from build123d import *

# Parameters (mm, degrees)
SKETCH1_R           = 32.5
SKETCH1_R_2         = 29.5
BOSS_EXTRUDE1_DEPTH = 72
BOSS_EXTRUDE2_DEPTH = 72
CIRPATTERN1_COUNT   = 3
CIRPATTERN1_ANGLE   = 120
SKETCH7_R           = 12.5
BOSS_EXTRUDE5_DEPTH = 72
SKETCH9_R           = 9.9
CUT_EXTRUDE4_DEPTH  = 86.419552797


with BuildPart() as part:
    # Sketch1 → Boss-Extrude1 (new body)
    with BuildSketch(Plane.XY):
        Circle(SKETCH1_R)
        Circle(SKETCH1_R_2, mode=Mode.SUBTRACT)
    extrude(amount=BOSS_EXTRUDE1_DEPTH)

    # Sketch2 → Boss-Extrude2 (add, through all)
    with BuildSketch(Plane.XY):
        with BuildLine():
            Line((-29.461839725, -1.5), (29.461839725, -1.5))
            ThreePointArc((29.461839725, -1.5), (29.5, 0), (29.461839725, 1.5))
            Line((29.461839725, 1.5), (-29.461839725, 1.5))
            ThreePointArc((-29.461839725, 1.5), (-29.5, 0), (-29.461839725, -1.5))
        make_face()
    boss_extrude2 = extrude(amount=BOSS_EXTRUDE2_DEPTH)

    # CirPattern1: Boss-Extrude2 ×3 about axis
    cirpattern1_axis = Axis((0, 0, 0), (0, 0, 1))
    for i in range(1, CIRPATTERN1_COUNT):
        add(boss_extrude2.rotate(cirpattern1_axis, i * CIRPATTERN1_ANGLE / (CIRPATTERN1_COUNT - 1)))

    # Sketch7 → Boss-Extrude5 (add, through all)
    with BuildSketch(Plane.XY):
        Circle(SKETCH7_R)
    extrude(amount=BOSS_EXTRUDE5_DEPTH)

    # Sketch9 → Cut-Extrude4 (cut, through all)
    with BuildSketch(Plane.XY):
        Circle(SKETCH9_R)
    extrude(amount=CUT_EXTRUDE4_DEPTH, mode=Mode.SUBTRACT)


solid = part.part
Geometry: final body of the model. Coordinates: model frame, mm. Give positions to 0.01 mm unless a question says otherwise; leave off trailing zeros. Loops run counter-clockwise (first coordinate to the right, second up) from the corner with the lowest first, then second, coordinate; pieces in that order, holes last. Notation, with made-up numbers: (75.25, -27.5) -> (100.25, -27.5) arc R30 ccw to (100.25, 2.5) -> close; hole circle Ø11 at (84.25, 15.25). An arc over 180 degrees is marked (long way). Put each result on its own line as item: value.
1. Pin query (flat end, axial travel): P1, Ø4, axis at x = -21, z = 62.5, coming from the +Y side; P2, Ø1.5, axis at x = -20, z = 31.5, coming from the +Y side; P3, Ø12, axis at y = -15, z = 54.5, coming from the -X side. Return the tip coordinate at first contact, or that it passes through.
Taken from the geometry:
P1: stops at y = 26.37
P2: stops at y = 26.19
P3: stops at x = -31.23
2. Pull-direction query (X, two-part tool) for faces 1 (the flat face through (-11.827, 17.484, 35.496)), 2 (the flat face through (-10, -3, 0)), 3 (the cylindrical face through (31, 9.76, 35.5)); classes: released by +X, released by -X, zero draft, split by the parting line, or undercut.
Taken from the geometry:
face 1: undercut
face 2: zero draft
face 3: split by the parting line
3. Cut plane A-A (y = 15). Return the cut outline in (x, z).
Taken from the geometry:
outline: (-28.83, 0) -> (-25.4, 0) -> (-25.4, 72) -> (-28.83, 72) -> close; (-10.39, 0) -> (-6.93, 0) -> (-6.93, 72) -> (-10.39, 72) -> close; (6.93, 0) -> (10.39, 0) -> (10.39, 72) -> (6.93, 72) -> close; (25.4, 0) -> (28.83, 0) -> (28.83, 72) -> (25.4, 72) -> close
4. Cut plane B-B (x = 0). Return the cut outline in (y, z), plus the area to 3 significant figures.
Taken from the geometry:
outline: (-32.5, 0) -> (-29.5, 0) -> (-29.5, 72) -> (-32.5, 72) -> close; (-12.5, 0) -> (-9.9, 0) -> (-9.9, 72) -> (-12.5, 72) -> close; (9.9, 0) -> (12.5, 0) -> (12.5, 72) -> (9.9, 72) -> close; (29.5, 0) -> (32.5, 0) -> (32.5, 72) -> (29.5, 72) -> close
area: 806 mm2
5. Cut plane D-D (x = -21.5). Return the cut outline in (y, z).
Taken from the geometry:
outline: (-24.37, 0) -> (-20.2, 0) -> (-20.2, 72) -> (-24.37, 72) -> close; (-1.5, 0) -> (1.5, 0) -> (1.5, 72) -> (-1.5, 72) -> close; (20.2, 0) -> (24.37, 0) -> (24.37, 72) -> (20.2, 72) -> close
6. Cut plane C-C (z = 65). Return the cut outline in (x, y), plus the area to 3 significant figures.
Taken from the geometry:
outline: circle Ø65 at (0, 0); hole (-29.46, -1.5) arc R29.5 ccw to (-16.03, -24.76) -> (-7.5, -10) arc R12.5 cw to (-12.41, -1.5) -> close; hole (-29.46, 1.5) -> (-12.41, 1.5) arc R12.5 cw to (-7.5, 10) -> (-16.03, 24.76) arc R29.5 ccw to start; hole (-13.43, -26.26) arc R29.5 ccw to (13.43, -26.26) -> (4.91, -11.5) arc R12.5 cw to (-4.91, -11.5) -> close; hole (-13.43, 26.26) -> (-4.91, 11.5) arc R12.5 cw to (4.91, 11.5) -> (13.43, 26.26) arc R29.5 ccw to start; hole circle Ø19.8 at (0, 0); hole (7.5, -10) -> (16.03, -24.76) arc R29.5 ccw to (29.46, -1.5) -> (12.41, -1.5) arc R12.5 cw to start; hole (7.5, 10) arc R12.5 cw to (12.41, 1.5) -> (29.46, 1.5) arc R29.5 ccw to (16.03, 24.76) -> close
area: 1,070 mm2
7. Ray query, line 1 along X through (y, z) = (-18, 41); line 2 along Y through (x, z) = (17, 23); line 3 along X through (y, z) = (-24.5, 58). Return the intervals inside material, ascending. Write a range as [from, to].
Taken from the geometry:
line 1: x = [-27.06, -23.37], [-12.12, -8.66], [8.66, 12.12], [23.37, 27.06]
line 2: y = [-27.7, -24.11], [-1.5, 1.5], [24.11, 27.7]
line 3: x = [-21.35, -16.43], [-15.88, -12.41], [12.41, 15.88], [16.43, 21.35]
